Could you check a few things on this model? Use its own coordinates, in mm. A direction names the side the tool comes from. Round coordinates to 2 decimals unless told otherwise and drop trailing zeros. Loops run counter-clockwise (first coordinate to the right, second up) from the corner with the lowest first, then second, coordinate; pieces in that order, holes last. Notation, with made-up numbers: (48.5, 23) -> (81.5, 23) arc R30 ccw to (81.5, 62) -> close; hole circle Ø8 at (53.5, 20.5). An arc over 180 degrees is marked (long way). One line per item, written item: value.
```python
from build123d import *

# Parameters (mm, degrees)
F0_R     = 38.1
F1_DEPTH = 6.35
F2_R     = 25.4
F3_DEPTH = 25.4
F4_R     = 38.1
F4_R_2   = 25.4
F5_DEPTH = 6.35
F6_R     = 3.175
F7_DEPTH = 38.101


with BuildPart() as f1:
    # F0 (on Front) → F1 (new body)
    with BuildSketch(Plane.XZ):
        Circle(F0_R)
    extrude(amount=F1_DEPTH)

    # F2 (on face) → F3 (join)
    with BuildSketch(Plane.XZ.offset(6.35)):
        Circle(F2_R)
    extrude(amount=F3_DEPTH)

    # F4 (on face) → F5 (join)
    with BuildSketch(Plane.XZ.offset(31.75)):
        Circle(F4_R)
        Circle(F4_R_2, mode=Mode.SUBTRACT)
        Circle(F4_R_2)
    extrude(amount=F5_DEPTH)

    # F6 (on face) → F7 (cut, through all)
    with BuildSketch(Plane.XZ.offset(38.1)):
        Circle(F6_R)
    extrude(amount=-F7_DEPTH, mode=Mode.SUBTRACT)


solid = f1.part
```
Item 1: If we section it at C-C on y = -16.5: List the corners of the cut face in (x, z) for me (3 decimals), plus the area to 3 significant figures.
Output:
outline: circle Ø50.8 at (0, 0); hole circle Ø6.35 at (0, 0)
area: 2,000 mm²
Item 2: If we section it at B-B on x = 0: List the corners of the cut face in (y, z) for me (3 decimals), plus the area to 3 significant figures.
Output:
outline: (-38.1, -38.1) -> (-31.75, -38.1) -> (-31.75, -25.4) -> (-6.35, -25.4) -> (-6.35, -38.1) -> (0, -38.1) -> (0, -3.175) -> (-38.1, -3.175) -> close; (-38.1, 3.175) -> (0, 3.175) -> (0, 38.1) -> (-6.35, 38.1) -> (-6.35, 25.4) -> (-31.75, 25.4) -> (-31.75, 38.1) -> (-38.1, 38.1) -> close
area: 2,020 mm²
Item 3: I need wall thicknesses on line 1 (Z direction, x = 0, y = -19.5) (3 decimals); line 2 (Y direction, x = 22, z = -31); line 3 (X direction, y = -23, z = -2). Which ranges of each line are inside material? Lowest first, please. Write a range as from..to.
Output:
line 1: z = -25.4..-3.175, 3.175..25.4
line 2: y = -38.1..-31.75, -6.35..0
line 3: x = -25.32..-2.47, 2.47..25.32
Item 4: For faces 4 (the face through (8, -31.75, -25)), 5 (the face through (8, -38.1, 1)), which set-ups out of +Z, -Z, +X, -X, +Y, -Y let a thin tool reach every point of the face, with its end or its side?
Output:
face 4: none
face 5: +Z, -Z, +X, -X, -Y
Item 5: Will these pins go through, and if not, where does the flat tip stop? pin 1 Ø4 at (x, y) = (3.5, -12.5) entering from -Z; pin 2 Ø1 at (x, y) = (8, -14) entering from +Z; pin 3 Ø2 at (x, y) = (18.5, -22) entering from +Z; pin 4 Ø5.5 at (x, z) = (0, 0) entering from -Y.
Output:
pin 1: stops at z = -25.36
pin 2: stops at z = 24.27
pin 3: stops at z = 18.41
pin 4: passes through
Item 6: If we mould it in two halves opening along Y, with no side actions, what happens to faces 1 (the face through (-5.506, -18.872, -24.796)), 2 (the face through (-0.69, -19.32, -3.1)), 3 (the face through (8, 0, 1))? For each: released by +Y, released by -Y, zero draft, split by the parting line, or undercut.
Output:
face 1: undercut
face 2: zero draft
face 3: released by +Y
Item 7: If we section it at A-A on z = 0: List the corners of the cut face in (x, y) for me (3 decimals), plus the area to 3 significant figures.
Output:
outline: (-38.1, -38.1) -> (-3.175, -38.1) -> (-3.175, 0) -> (-38.1, 0) -> (-38.1, -6.35) -> (-25.4, -6.35) -> (-25.4, -31.75) -> (-38.1, -31.75) -> close; (3.175, -38.1) -> (38.1, -38.1) -> (38.1, -31.75) -> (25.4, -31.75) -> (25.4, -6.35) -> (38.1, -6.35) -> (38.1, 0) -> (3.175, 0) -> close
area: 2,020 mm²
Item 8: If we section it at D-D on z = -13: List the corners of the cut face in (x, y) for me.
Output:
outline: (-35.81, -38.1) -> (35.81, -38.1) -> (35.81, -31.75) -> (21.82, -31.75) -> (21.82, -6.35) -> (35.81, -6.35) -> (35.81, 0) -> (-35.81, 0) -> (-35.81, -6.35) -> (-21.82, -6.35) -> (-21.82, -31.75) -> (-35.81, -31.75) -> close
